```python
from build123d import *

# Parameters (mm, degrees)
SKETCH1_W               = 76.2
SKETCH1_H               = 76.2
BOSS_EXTRUDE1_DEPTH     = 12.7
SKETCH2_R               = 33.3375
CUT_EXTRUDE1_DEPTH      = 10.16
SKETCH3_R               = 9.525
CUT_EXTRUDE2_DEPTH      = 19.05
CUT_EXTRUDE3_DEPTH      = 55.831064188
CUT_EXTRUDE3_DEPTH_BACK = 55.831064188
SKETCH4_R               = 1.27
SKETCH4_R_2             = 2.5527
F_10_32_TAPPED_HOLE1_D  = 4.0386
BOSS_EXTRUDE2_START     = 2.286
SKETCH7_W               = 76.2
SKETCH7_H               = 76.2
SKETCH7_R               = 2.5527
SKETCH7_R_2             = 2.0193
SKETCH7_R_3             = 9.525
BOSS_EXTRUDE2_DEPTH     = 2.286


with BuildPart() as part:
    # Sketch1 → Boss-Extrude1 (new body)
    with BuildSketch(Plane.XY):
        Rectangle(SKETCH1_W, SKETCH1_H)
    extrude(amount=BOSS_EXTRUDE1_DEPTH)

    # Sketch2 → Cut-Extrude1 (cut)
    with BuildSketch(Plane.XY.offset(12.7)):
        Circle(SKETCH2_R)
    extrude(amount=-CUT_EXTRUDE1_DEPTH, mode=Mode.SUBTRACT)

    # Sketch3 → Cut-Extrude2 (cut)
    with BuildSketch(Plane.XY.offset(2.54)):
        Circle(SKETCH3_R)
    extrude(amount=-CUT_EXTRUDE2_DEPTH, mode=Mode.SUBTRACT)

    # Sketch4 → Cut-Extrude3 (cut, two sides: drawn at the far end of the back side and taken through both)
    with BuildSketch(Plane.XY.offset(2.54).offset(-CUT_EXTRUDE3_DEPTH_BACK)):
        with Locations((-31.75, 31.75)):
            Circle(SKETCH4_R)
        with Locations((31.75, 31.75)):
            Circle(SKETCH4_R)
        with Locations((31.75, -31.75)):
            Circle(SKETCH4_R)
        with Locations((-31.75, -31.75)):
            Circle(SKETCH4_R)
        with Locations((-25.4, 0)):
            Circle(SKETCH4_R_2)
        with Locations((25.4, 0)):
            Circle(SKETCH4_R_2)
    extrude(amount=CUT_EXTRUDE3_DEPTH + CUT_EXTRUDE3_DEPTH_BACK, mode=Mode.SUBTRACT)

    # #10-32 Tapped Hole1 (through all)
    with Locations(Plane.XY.offset(12.7)):
        with Locations((-31.75, 31.75), (-31.75, -31.75), (31.75, -31.75), (31.75, 31.75)):
            Hole(F_10_32_TAPPED_HOLE1_D / 2)

    # Sketch7 → Boss-Extrude2 (add)
    with BuildSketch(Plane(origin=(0, 0, 0), x_dir=(-1, 0, 0), z_dir=(0, 0, -1)).offset(BOSS_EXTRUDE2_START)):
        Rectangle(SKETCH7_W, SKETCH7_H)
        with Locations(Location((-25.4, 0, 0), (0, 0, 180))):
            Circle(SKETCH7_R, mode=Mode.SUBTRACT)
        with Locations(Location((-31.75, 31.75, 0), (0, 0, 180))):
            Circle(SKETCH7_R_2, mode=Mode.SUBTRACT)
        with Locations(Location((0, 0, 0), (0, 0, 180))):
            Circle(SKETCH7_R_3, mode=Mode.SUBTRACT)
        with Locations(Location((25.4, 0, 0), (0, 0, 180))):
            Circle(SKETCH7_R, mode=Mode.SUBTRACT)
        with Locations(Location((31.75, 31.75, 0), (0, 0, 180))):
            Circle(SKETCH7_R_2, mode=Mode.SUBTRACT)
        with Locations(Location((31.75, -31.75, 0), (0, 0, 180))):
            Circle(SKETCH7_R_2, mode=Mode.SUBTRACT)
        with Locations(Location((-31.75, -31.75, 0), (0, 0, 180))):
            Circle(SKETCH7_R_2, mode=Mode.SUBTRACT)
    extrude(amount=-BOSS_EXTRUDE2_DEPTH)


solid = part.part
```
Geometry: final body of the model. Coordinates: model frame, mm. Give positions to 0.01 mm unless a question says otherwise; leave off trailing zeros. Write each loop counter-clockwise with the first axis right and the second up, starting at its lowest first coordinate (ties: lowest second). Pieces come first, ordered by that corner, then holes.
1. Section query C-C, the plane x = 0. Return loops of the section in (y, z) (1 decimal), then the cut area to 3 significant figures.
2. Draft query along Y for faces 1 (the flat face through (1, 38.1, 5)), 2 (the flat face through (7, -7, 2.54)), 3 (the cylindrical face through (31.8, 10.01, 7.69)), 4 (the flat face through (-38.1, -1, 5)). Return one class per face: released by +Y, released by -Y, zero draft, split by the parting line, or undercut.
3. Section query D-D, the plane y = 31.75. Return loops of the section in (x, z), then the cut area to 3 significant figures.
4. Section query B-B, the plane z = 8.75. Count the separate pieces of the cut face and the enclosed holes in it, then the cut area to 3 significant figures.
5. Pin query (flat end, axial travel): P1, Ø5.5, axis at x = -31.75, y = 31.75, coming from the -Z side; P2, Ø22, axis at x = 0, y = 0, coming from the +Z side. Return the tip coordinate at first contact, or that it passes through.
6. Section query A-A, the plane y = 0. Return loops of the section in (x, z) (1 decimal).
7. Line query: probe 1 along Y at (x, z) = (31.75, -0.65); probe 2 along Y at (x, z) = (25.4, 0.95). Output: solid intervals per line, ascending.
Computed:
1. outline: (-38.1, -2.3) - (-9.5, -2.3) - (-9.5, 2.5) - (-33.3, 2.5) - (-33.3, 12.7) - (-38.1, 12.7) - close; (9.5, -2.3) - (38.1, -2.3) - (38.1, 12.7) - (33.3, 12.7) - (33.3, 2.5) - (9.5, 2.5) - close
1. area: 373 mm2
2. face 1: released by +Y
2. face 2: undercut
2. face 3: undercut
2. face 4: zero draft
3. outline: (-38.1, -2.29) - (-33.77, -2.29) - (-33.77, 12.7) - (-38.1, 12.7) - close; (-29.73, -2.29) - (29.73, -2.29) - (29.73, 12.7) - (10.16, 12.7) - (10.16, 2.54) - (-10.16, 2.54) - (-10.16, 12.7) - (-29.73, 12.7) - close; (33.77, -2.29) - (38.1, -2.29) - (38.1, 12.7) - (33.77, 12.7) - close
3. area: 814 mm2
4. separate pieces: 1
4. enclosed holes: 5
4. area: 2,260 mm2
5. P1: stops at z = -2.29
5. P2: stops at z = 2.54
6. outline: (-38.1, -2.3) - (-28, -2.3) - (-28, 2.5) - (-33.3, 2.5) - (-33.3, 12.7) - (-38.1, 12.7) - close; (-22.8, -2.3) - (-9.5, -2.3) - (-9.5, 2.5) - (-22.8, 2.5) - close; (9.5, -2.3) - (22.8, -2.3) - (22.8, 2.5) - (9.5, 2.5) - close; (28, -2.3) - (38.1, -2.3) - (38.1, 12.7) - (33.3, 12.7) - (33.3, 2.5) - (28, 2.5) - close
7. probe 1: y = -38.1 to -33.77, -29.73 to 29.73, 33.77 to 38.1
7. probe 2: y = -38.1 to -2.55, 2.55 to 38.1
